For this review, use the dimensioned drawing (mm, ordinates from the lowest corner) and the shaded views. Coordinates: 2 decimals unless noted, no trailing zeros. Loops run counter-clockwise (first coordinate to the right, second up) from the corner with the lowest first, then second, coordinate; pieces in that order, holes last. Notation, with made-up numbers: M 42,66 L 46,66 A30 cw 46,100 Z; hole C 59,7 d9. An arc over 180 degrees is marked long. Use CSV: the item, a comma, the result in double quotes. Start each with the question number.
1. Add section A-A, the plane x = 4.25. Write out the cut boundary in (y, z), then the cut area to 3 significant figures.
2. Add section C-C, the plane y = 1.05. Write out the cut boundary in (x, z), then the cut area to 3 significant figures.
3. Add section B-B, the plane z = 18.5. Write out the cut boundary in (x, y), then the cut area to 3 significant figures.
4. For L1, parallel to Z at x = 4.25, y = 0.55; L2, parallel to X at y = 1.25, z = 22; L3, parallel to Y at x = 44.5, z = 5.75, list the stretches that pass through material, from the lowest coordinate up.
5. Add section D-D, the plane x = 34.5. Write out the cut boundary in (y, z), then the cut area to 3 significant figures.
6. Clearance check with flat-ended pins moving along their axes: P1, Ø4, axis at x = 40.5, z = 17, coming from the +Y side; P2, Ø1.3, axis at y = 3, z = 17.5, coming from the +X side; P3, Ø2.5, axis at x = 4.25, z = 22.5, coming from the -Y side; P4, Ø2, axis at x = 34, y = 3, coming from the +Z side. State where each tip first meets the part, or that it passes through.
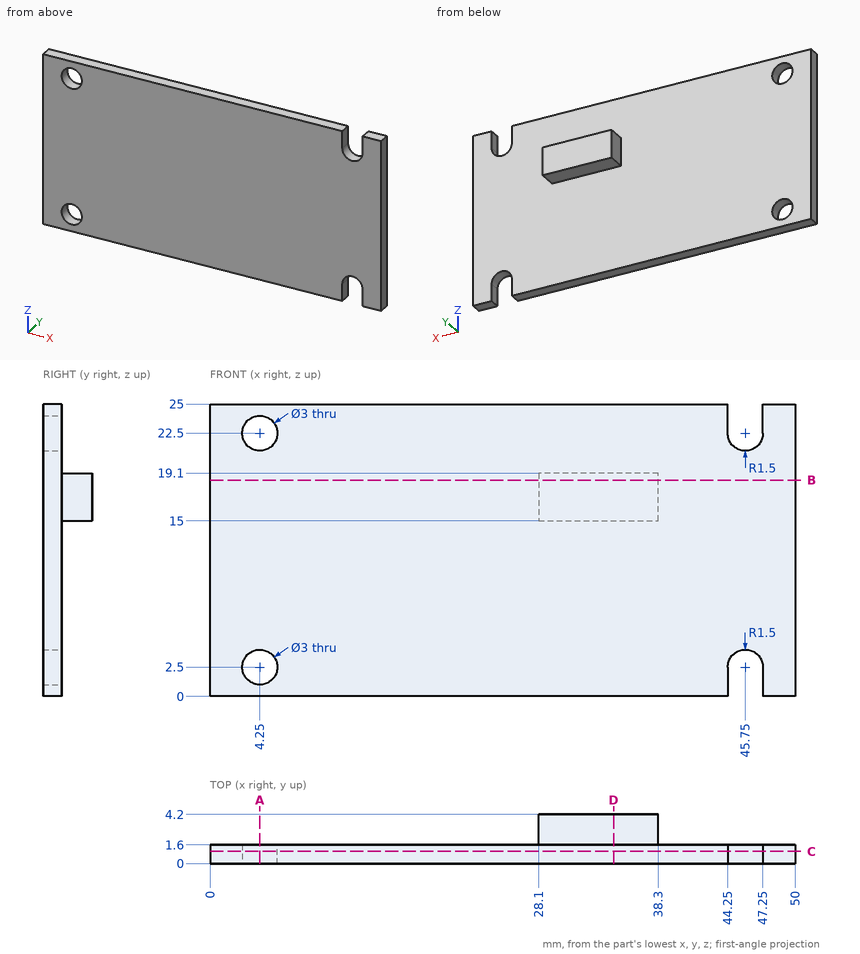
Computed:
1,outline,"M 0,0 L 1.6,0 L 1.6,1 L 0,1 Z; M 0,4 L 1.6,4 L 1.6,21 L 0,21 Z; M 0,24 L 1.6,24 L 1.6,25 L 0,25 Z"
1,area,"30.4 mm^2"
2,outline,"M 0,0 L 44.25,0 L 44.25,2.5 A1.5 cw 47.25,2.5 L 47.25,0 L 50,0 L 50,25 L 47.25,25 L 47.25,22.5 A1.5 cw 44.25,22.5 L 44.25,25 L 0,25 Z; hole C 4.25,2.5 d3; hole C 4.25,22.5 d3"
2,area,"1,210 mm^2"
3,outline,"M 0,0 L 50,0 L 50,1.6 L 38.3,1.6 L 38.3,4.2 L 28.1,4.2 L 28.1,1.6 L 0,1.6 Z"
3,area,"107 mm^2"
4,L1,"z = 0 to 1, 4 to 21, 24 to 25"
4,L2,"x = 0 to 2.84, 5.66 to 44.34, 47.16 to 50"
4,L3,"y = 0 to 1.6"
5,outline,"M 0,0 L 1.6,0 L 1.6,15 L 4.2,15 L 4.2,19.1 L 1.6,19.1 L 1.6,25 L 0,25 Z"
5,area,"50.7 mm^2"
6,P1,"stops at y = 1.6"
6,P2,"stops at x = 38.3"
6,P3,"passes through"
6,P4,"stops at z = 19.1"
